Here's how the part is built. I have some questions about the finished solid (model axes, mm). Face numbers are marked on the shaded views. Coordinates: 2 decimals unless noted, no trailing zeros. Write each loop counter-clockwise with the first axis right and the second up, starting at its lowest first coordinate (ties: lowest second). Pieces come first, ordered by that corner, then holes.
(1) For pin 1 Ø11 at (y, z) = (-49.21, -1.52) entering from +X, with a flat end and sliding along its axis, tell me the tip position at first contact or that it passes through.
(2) Please list where these lines run through material, in increasing order: probe 1 along Y at (x, z) = (-3, -3.5); probe 2 along Y at (x, z) = (0.75, -5); probe 3 along Y at (x, z) = (3, 17).
(3) Imagine slicing it at D-D, the plane y = 54. List the corners of the cut face in (x, z) for me.
(4) Imagine slicing it at C-C, the plane z = 3. List the corners of the cut face in (x, y) for me.
(5) Imagine slicing it at A-A, the plane z = 19. List the corners of the cut face in (x, y) for me, plus the area to 3 significant figures.
(6) Thinking about a two-plate mould opening in Y: for the marked faces 1, 2, 3 and 4, which applies, released by +Y, released by -Y, zero draft, split by the parting line, or undercut?
(7) Imagine slicing it at B-B, the plane x = -1. List the corners of the cut face in (y, z) for me (3 decimals), plus the area to 3 significant figures.
```python
from build123d import *

# Parameters (mm, degrees)
SKETCH1_W           = 16.2814
SKETCH1_H           = 177.8
BOSS_EXTRUDE1_DEPTH = 25.4
SKETCH2_R           = 6.75767
CUT_EXTRUDE1_DEPTH  = 94.879997795
SKETCH3_R           = 8.7641176
CUT_EXTRUDE2_DEPTH  = 11.3284
CUT_EXTRUDE3_DEPTH  = 9.525
FILLET1_R           = 2.54


with BuildPart() as part:
    # Sketch1 → Boss-Extrude1 (new, symmetric)
    with BuildSketch(Plane.XY):
        Rectangle(SKETCH1_W, SKETCH1_H)
    extrude(amount=BOSS_EXTRUDE1_DEPTH, both=True)

    # Sketch2 → Cut-Extrude1 (cut, through all)
    with BuildSketch(Plane(origin=(8.1407, 0, 0), x_dir=(0, 0, -1), z_dir=(1, 0, 0))):
        with Locations((1.524, 49.211738)):
            Circle(SKETCH2_R)
        with Locations((1.524, -49.211738)):
            Circle(SKETCH2_R)
    extrude(amount=-CUT_EXTRUDE1_DEPTH, mode=Mode.SUBTRACT)

    # Sketch3 → Cut-Extrude2 (cut)
    with BuildSketch(Plane(origin=(8.1407, 0, 0), x_dir=(0, 0, -1), z_dir=(1, 0, 0))):
        with Locations((1.524, 49.211738)):
            Circle(SKETCH3_R)
        with Locations((1.524, -49.211738)):
            Circle(SKETCH3_R)
    extrude(amount=-CUT_EXTRUDE2_DEPTH, mode=Mode.SUBTRACT)

    # Sketch5 → Cut-Extrude3 (cut)
    with BuildSketch(Plane.XY.offset(25.4)):
        with BuildLine():
            Line((1.3843, 24.702073714), (8.1407, 27.901182182))
            Line((8.1407, 27.901182182), (8.1407, 0.236876892))
            Line((8.1407, 0.236876892), (5.147798748, 0.634218973))
            ThreePointArc((5.147798748, 0.634218973), (-5.728317972, 11.261694019), (1.3843, 24.702073714))
        make_face()
    extrude(amount=-CUT_EXTRUDE3_DEPTH, mode=Mode.SUBTRACT)

    # Fillet1
    fillet1_edges = [part.edges().sort_by_distance(p)[0] for p in [
        (8.1407, 27.901182182, 20.6375),
        (8.1407, 0.236876892, 20.6375),
    ]]
    fillet(fillet1_edges, radius=FILLET1_R)


solid = part.part
```
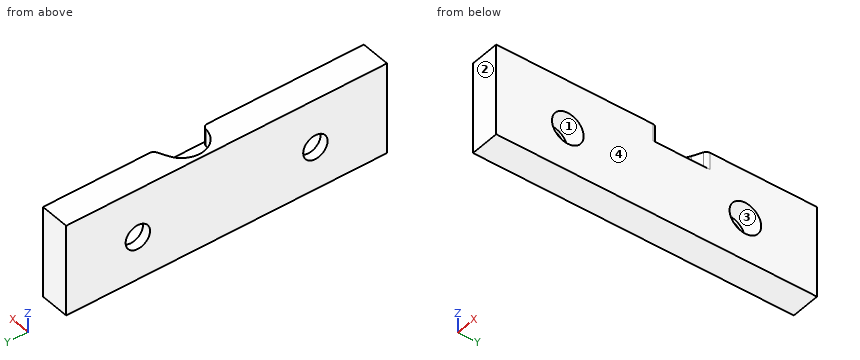
Recorded:
1. pin 1: passes through
2. probe 1: y = -88.9 to -57.75, -40.67 to 40.67, 57.75 to 88.9
2. probe 2: y = -88.9 to -57.26, -41.17 to 41.17, 57.26 to 88.9
2. probe 3: y = -88.9 to 1.11, 25.47 to 88.9
3. outline: (-8.14, -25.4) - (8.14, -25.4) - (8.14, -8.86) - (-3.19, -8.86) - (-3.19, -6.29) - (-8.14, -6.29) - close; (-8.14, 3.24) - (-3.19, 3.24) - (-3.19, 5.82) - (8.14, 5.82) - (8.14, 25.4) - (-8.14, 25.4) - close
4. outline: (-8.14, -88.9) - (8.14, -88.9) - (8.14, -56.72) - (-3.19, -56.72) - (-3.19, -54.23) - (-8.14, -54.23) - close; (-8.14, -44.19) - (-3.19, -44.19) - (-3.19, -41.71) - (8.14, -41.71) - (8.14, 41.71) - (-3.19, 41.71) - (-3.19, 44.19) - (-8.14, 44.19) - close; (-8.14, 54.23) - (-3.19, 54.23) - (-3.19, 56.72) - (8.14, 56.72) - (8.14, 88.9) - (-8.14, 88.9) - close
5. outline: (-8.14, -88.9) - (8.14, -88.9) - (8.14, -1.99) arc R2.54 ccw to (5.93, 0.53) - (5.15, 0.63) arc R12.7 cw to (1.38, 24.7) - (6.69, 27.21) arc R2.54 ccw to (8.14, 29.51) - (8.14, 88.9) - (-8.14, 88.9) - close
5. area: 2,600 mm2
6. face 1: undercut
6. face 2: released by -Y
6. face 3: undercut
6. face 4: zero draft
7. outline: (-88.9, -25.4) - (88.9, -25.4) - (88.9, 25.4) - (23.231, 25.4) - (23.231, 15.875) - (3.216, 15.875) - (3.216, 25.4) - (-88.9, 25.4) - close; hole circle Ø17.528 at (-49.212, -1.524); hole circle Ø17.528 at (49.212, -1.524)
7. area: 8,360 mm2
